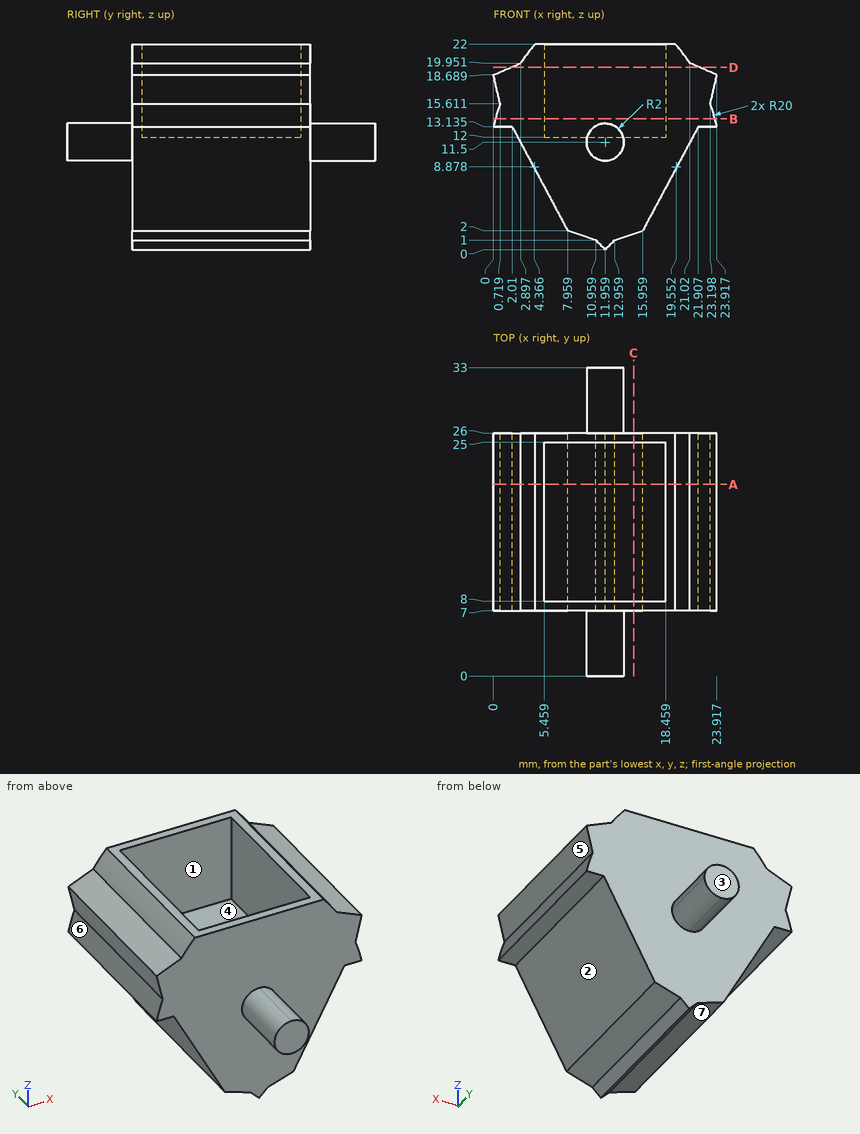
Job drawing, mm, ordinate dimensions from the low corner. One solid piece. A direction names the side the tool comes from. Coordinates: 2 decimals unless noted, no trailing zeros. Write each loop counter-clockwise with the first axis right and the second up, starting at its lowest first coordinate (ties: lowest second). Pieces come first, ordered by that corner, then holes.
Item 1: Slice it at A-A (y = 20.5). Write the cut outline in (x, z) (1 decimal).
Item 2: Mould opens along X. For the marked faces 1, 2 and 3 say: released by +X, released by -X, zero draft, split by the parting line, or undercut.
Item 3: Slice it at D-D (z = 19.5). Write the cut outline in (x, y) (1 decimal).
Item 4: Pin check, flat tips, straight feed: pin 1 (4 mm diameter, centred on x = 15, z = 7, fed in from -Y); pin 2 (4 mm diameter, centred on y = 17, z = 3, fed in from -X) (1 decimal); pin 3 (2 mm diameter, centred on y = 17.5, z = 14.5, fed in from +X) (1 decimal). Stop position of each tip, or through.
Item 5: Probe line 1 (Y direction, x = 9, z = 20.75); line 2 (Y direction, x = 20, z = 15.25); line 3 (X direction, y = 12.5, z = 13) (1 decimal). List the from-to ranges inside material, lowest first.
Item 6: Slice it at B-B (z = 14). Write the cut outline in (x, y), and give its area (3 significant figures).
Item 7: Slice it at C-C (x = 15). Write the cut outline in (y, z).
Item 8: Which spindle directions (+Z, -Z, +X, -X, +Y, -Y) get a long thin tool onto all of the face, cutting with end or side? Do the marked faces 4, 5, 6 and 7. Say none if no direction does.
Results found:
1. outline: (0, 13.1) - (2, 13.1) - (8, 2) - (11, 1) - (12, 0) - (13, 1) - (16, 2) - (21.9, 13.1) - (23.9, 13.1) arc R20 ccw to (23.2, 15.6) - (23.9, 18.7) - (21, 20) arc R20 ccw to (19.5, 22) - (18.5, 22) - (18.5, 12) - (5.5, 12) - (5.5, 22) - (4.5, 22) arc R20 ccw to (2.9, 20) - (0, 18.7) - (0.7, 15.6) arc R20 ccw to start
2. face 1: undercut
2. face 2: released by +X
2. face 3: zero draft
3. outline: (1.9, 7) - (22.1, 7) - (22.1, 26) - (1.9, 26) - close; hole (5.5, 8) - (18.5, 8) - (18.5, 25) - (5.5, 25) - close
4. pin 1: stops at y = 7
4. pin 2: stops at x = 6.4
4. pin 3: stops at x = 23.8
5. line 1: y = 7 to 8, 25 to 26
5. line 2: y = 7 to 26
5. line 3: x = 2.1 to 5.5, 18.5 to 21.8
6. outline: (0.22, 7) - (23.7, 7) - (23.7, 26) - (0.22, 26) - close; hole (5.46, 8) - (18.46, 8) - (18.46, 25) - (5.46, 25) - close
6. area: 225 mm2
7. outline: (7, 1.68) - (26, 1.68) - (26, 22) - (25, 22) - (25, 12) - (8, 12) - (8, 22) - (7, 22) - close
8. face 4: +Z
8. face 5: +X, +Y, -Y
8. face 6: -X, +Y, -Y
8. face 7: -Z, -X, +Y, -Y
